```python
from build123d import *

# Parameters (mm, degrees)
SKETCH1_W            = 208
SKETCH1_H            = 128
SKETCH1_W_2          = 200
SKETCH1_H_2          = 120
SKETCH1_W_3          = 8
SKETCH1_H_3          = 8
BOSS_EXTRUDE1_DEPTH  = 16
SKETCH1_3_W          = 208
SKETCH1_3_H          = 128
SKETCH1_3_R          = 8.4
BOSS_EXTRUDE2_DEPTH  = 4
M4_CLEARANCE_HOLE1_D = 4.8
FILLET2_R            = 8
FILLET1_R            = 4
FILLET3_R            = 8
FILLET4_R            = 3
SKETCH8_R            = 4.25
CUT_EXTRUDE1_DEPTH   = 7


# Some blends are built 0.0001 mm under size
with BuildPart() as part:
    # Sketch1 → Boss-Extrude1 (new body)
    # profile 1 of 5: a face of its own
    with BuildSketch(Plane(origin=(0, 0, 0), x_dir=(1, 0, 0), z_dir=(0, 1, 0))):
        with Locations((100, 60)):
            Rectangle(SKETCH1_W, SKETCH1_H)
        with Locations((100, 60)):
            Rectangle(SKETCH1_W_2, SKETCH1_H_2, mode=Mode.SUBTRACT)
    # profile 2 of 5: a face of its own
    with BuildSketch(Plane(origin=(0, 0, 0), x_dir=(1, 0, 0), z_dir=(0, 1, 0))):
        with Locations((4, 4)):
            Rectangle(SKETCH1_W_3, SKETCH1_H_3)
    # profile 3 of 5: a face of its own
    with BuildSketch(Plane(origin=(0, 0, 0), x_dir=(1, 0, 0), z_dir=(0, 1, 0))):
        with Locations((196, 4)):
            Rectangle(SKETCH1_W_3, SKETCH1_H_3)
    # profile 4 of 5: a face of its own
    with BuildSketch(Plane(origin=(0, 0, 0), x_dir=(1, 0, 0), z_dir=(0, 1, 0))):
        with Locations((196, 116)):
            Rectangle(SKETCH1_W_3, SKETCH1_H_3)
    # profile 5 of 5: a face of its own
    with BuildSketch(Plane(origin=(0, 0, 0), x_dir=(1, 0, 0), z_dir=(0, 1, 0))):
        with Locations((4, 116)):
            Rectangle(SKETCH1_W_3, SKETCH1_H_3)
    extrude(amount=-BOSS_EXTRUDE1_DEPTH)

    # Sketch1<3> → Boss-Extrude2 (add)
    with BuildSketch(Plane(origin=(0, 0, 0), x_dir=(1, 0, 0), z_dir=(0, 1, 0))):
        with Locations((100, 60)):
            Rectangle(SKETCH1_3_W, SKETCH1_3_H)
        with Locations(Location((85, 90, 0), (0, 0, 270))):
            Circle(SKETCH1_3_R, mode=Mode.SUBTRACT)
        with Locations(Location((19.5, 100.5, 0), (0, 0, 270))):
            Circle(SKETCH1_3_R, mode=Mode.SUBTRACT)
        with Locations(Location((19.5, 19.5, 0), (0, 0, 270))):
            Circle(SKETCH1_3_R, mode=Mode.SUBTRACT)
        with Locations(Location((19.5, 46.5, 0), (0, 0, 270))):
            Circle(SKETCH1_3_R, mode=Mode.SUBTRACT)
        with Locations(Location((85, 30, 0), (0, 0, 270))):
            Circle(SKETCH1_3_R, mode=Mode.SUBTRACT)
        with Locations(Location((85, 60, 0), (0, 0, 270))):
            Circle(SKETCH1_3_R, mode=Mode.SUBTRACT)
        with Locations(Location((149, 19.5, 0), (0, 0, 270))):
            Circle(SKETCH1_3_R, mode=Mode.SUBTRACT)
        with Locations(Location((181, 19.5, 0), (0, 0, 270))):
            Circle(SKETCH1_3_R, mode=Mode.SUBTRACT)
        with BuildLine():
            ThreePointArc((163.25, 48.633932078), (153.5, 60), (163.25, 71.366067922))
            Line((163.25, 71.366067922), (163.25, 72.25))
            ThreePointArc((163.25, 72.25), (165, 74), (166.75, 72.25))
            Line((166.75, 72.25), (166.75, 71.366067922))
            ThreePointArc((166.75, 71.366067922), (176.5, 60), (166.75, 48.633932078))
            Line((166.75, 48.633932078), (166.75, 47.75))
            ThreePointArc((166.75, 47.75), (165, 46), (163.25, 47.75))
            Line((163.25, 47.75), (163.25, 48.633932078))
        make_face(mode=Mode.SUBTRACT)
        with Locations(Location((19.5, 73.5, 0), (0, 0, 270))):
            Circle(SKETCH1_3_R, mode=Mode.SUBTRACT)
    extrude(amount=BOSS_EXTRUDE2_DEPTH)

    # M4 Clearance Hole1 (through all)
    with Locations(Plane(origin=(0, 4, 0), x_dir=(1, 0, 0), z_dir=(0, 1, 0))):
        with Locations((3, 117), (197, 3), (3, 3), (197, 117)):
            Hole(M4_CLEARANCE_HOLE1_D / 2)

    # Fillet2
    fillet2_edges = [part.edges().sort_by_distance(p)[0] for p in [
        (204, -6, 4),
        (-4, -6, 4),
        (-4, -6, -124),
        (204, -6, -124),
    ]]
    fillet(fillet2_edges, radius=FILLET2_R)

    # Fillet1
    fillet1_edges = [part.edges().sort_by_distance(p)[0] for p in [
        (192, -8, 0),
        (192, -8, -8),
        (200, -8, -8),
        (8, -8, 0),
        (8, -8, -8),
        (0, -8, -8),
        (0, -8, -112),
        (8, -8, -120),
        (8, -8, -112),
        (192, -8, -120),
        (192, -8, -112),
        (200, -8, -112),
    ]]
    fillet(fillet1_edges, radius=FILLET1_R - 0.0001)  # a hair under: the kernel refuses the full size

    # Fillet3
    # the kernel refuses this fillet: 8 mm, written as the material it takes off along each edge
    with BuildSketch(Plane(origin=(-4, 4, -116), x_dir=(0, -1, 0), z_dir=(0, 0, 1)), Plane(origin=(204, 4, -4), x_dir=(0, -1, 0), z_dir=(0, 0, -1))) as fillet3_piece_1:
        with BuildLine():
            CenterArc((FILLET3_R, FILLET3_R), FILLET3_R, 180, 90)
            Line((0, FILLET3_R), (0, 0))
            Line((0, 0), (FILLET3_R, 0))
        make_face()
    extrude(amount=112, mode=Mode.SUBTRACT)
    with BuildSketch(Plane(origin=(196, 4, -124), x_dir=(0, -1, 0), z_dir=(-1, 0, 0)), Plane(origin=(4, 4, 4), x_dir=(0, -1, 0), z_dir=(1, 0, 0))) as fillet3_piece_2:
        with BuildLine():
            CenterArc((FILLET3_R, FILLET3_R), FILLET3_R, 180, 90)
            Line((0, FILLET3_R), (0, 0))
            Line((0, 0), (FILLET3_R, 0))
        make_face()
    extrude(amount=192, mode=Mode.SUBTRACT)
    with BuildSketch(Plane(origin=(4, 4, -4), x_dir=(0, 0, 1), z_dir=(1, 0, 0))) as fillet3_piece_3:
        with BuildLine():
            CenterArc((8 - FILLET3_R, FILLET3_R), FILLET3_R, 270, 90)
            Line((8 - FILLET3_R, 0), (8, 0))
            Line((8, 0), (8, FILLET3_R))
        make_face()
    revolve(axis=Axis((4, 4, -4), (0, -1, 0)), revolution_arc=90, mode=Mode.SUBTRACT)
    with BuildSketch(Plane(origin=(196, 4, -4), x_dir=(1, 0, 0), z_dir=(0, 0, -1))) as fillet3_piece_4:
        with BuildLine():
            CenterArc((8 - FILLET3_R, FILLET3_R), FILLET3_R, 270, 90)
            Line((8 - FILLET3_R, 0), (8, 0))
            Line((8, 0), (8, FILLET3_R))
        make_face()
    revolve(axis=Axis((196, 4, -4), (0, -1, 0)), revolution_arc=90, mode=Mode.SUBTRACT)
    with BuildSketch(Plane(origin=(196, 4, -116), x_dir=(1, 0, 0), z_dir=(0, 0, 1))) as fillet3_piece_5:
        with BuildLine():
            CenterArc((8 - FILLET3_R, -FILLET3_R), FILLET3_R, 0, 90)
            Line((8 - FILLET3_R, 0), (8, 0))
            Line((8, 0), (8, -FILLET3_R))
        make_face()
    revolve(axis=Axis((196, 4, -116), (0, 1, 0)), revolution_arc=90, mode=Mode.SUBTRACT)
    with BuildSketch(Plane(origin=(4, 4, -116), x_dir=(0, 0, -1), z_dir=(1, 0, 0))) as fillet3_piece_6:
        with BuildLine():
            CenterArc((8 - FILLET3_R, -FILLET3_R), FILLET3_R, 0, 90)
            Line((8 - FILLET3_R, 0), (8, 0))
            Line((8, 0), (8, -FILLET3_R))
        make_face()
    revolve(axis=Axis((4, 4, -116), (0, 1, 0)), revolution_arc=90, mode=Mode.SUBTRACT)

    # Fillet4
    fillet4_edges = [part.edges().sort_by_distance(p)[0] for p in [
        (200, 0, -60),
        (100, 0, 0),
        (0, 0, -60),
        (100, 0, -120),
        (198.828456414, 0, -110.828456414),
        (190.828456414, 0, -118.828456414),
        (9.171543586, 0, -118.828456414),
        (1.171543586, 0, -110.828456414),
        (1.171543586, 0, -9.171543586),
        (9.171543586, 0, -1.171543586),
        (198.828456414, 0, -9.171543586),
        (190.828456414, 0, -1.171543586),
        (193.171543586, 0, -6.828456414),
        (6.828456414, 0, -6.828456414),
        (6.828456414, 0, -113.171543586),
        (193.171543586, 0, -113.171543586),
    ]]
    fillet(fillet4_edges, radius=FILLET4_R)

    # Sketch8 → Cut-Extrude1 (cut)
    with BuildSketch(Plane(origin=(0, 4, 0), x_dir=(1, 0, 0), z_dir=(0, 1, 0))):
        with Locations(Location((3, 117, 0), (0, 0, 270))):
            Circle(SKETCH8_R)
        with Locations(Location((197, 117, 0), (0, 0, 270))):
            Circle(SKETCH8_R)
        with Locations(Location((197, 3, 0), (0, 0, 270))):
            Circle(SKETCH8_R)
        with Locations(Location((3, 3, 0), (0, 0, 270))):
            Circle(SKETCH8_R)
    extrude(amount=-CUT_EXTRUDE1_DEPTH, mode=Mode.SUBTRACT)


solid = part.part
```
Geometry check sheet. Reference: the model listing, model coordinates, mm. A direction names the side the tool comes from. Coordinates: 2 decimals unless noted, no trailing zeros. Order: outer loops, then holes, each group sorted by start corner. A loop starts at its lowest first (then second) coordinate and runs counter-clockwise, first axis right, second up. Notation, with made-up numbers: M 18,57.25 L 25,57.25 A25 ccw 25,71.25 Z; hole C 77,51.25 d9. An arc over 180 degrees is marked long. One line per question, with ' | ' between items. Start each with the question number.
Item 1: Cross-section at C-C on x = 85. Enter the section's corners in (y, z).
Item 2: Set-up check for faces 1 (the cylindrical face through (153.5, 2, -59.8)), 2 (the cylindrical face through (-1.594, 1.719, -60.784)), 3 (the cylindrical face through (1.141, -9.591, -9.203)): record each of +Z, -Z, +X, -X, +Y, -Y from which the full face is reachable in a straight line by a thin tool's end or side.
Item 3: Cross-section at B-B on z = -90. Enter the section's corners in (x, y), then the cut area to 3 significant figures.
Item 4: Material ranges on L1, parallel to X at y = -9.5, z = -88.5; L2, parallel to Z at x = 158, y = -13.75; L3, parallel to Z at x = 3, y = 1, recorded low to high. Write a range as [from, to].
Item 5: Cross-section at A-A on x = 149. Enter the section's corners in (y, z), then the cut area to 3 significant figures.
Item 6: Cross-section at D-D on z = -60. Enter the section's corners in (x, y), then the cut area to 3 significant figures.
Item 7: Gauge pin test, flat ends, axial feed: pin 1 (8 mm diameter, centred on x = 126.5, z = -35, fed in from -Y); pin 2 (15 mm diameter, centred on x = 85, z = -90, fed in from -Y); pin 3 (10 mm diameter, centred on x = 176, y = 2, fed in from +Z); pin 4 (0.7 mm diameter, centred on y = 2.5, z = -48.5, fed in from -X). Record the tip position at first contact, or that the pin passes through.
Item 8: Draft check along X on faces 4 (the flat face through (99, -10, 4)), 5 (the cylindrical face through (-1.719, -9.916, 1.594)), 6 (the cylindrical face through (19.87, 1.97, -54.89)), 7 (the cylindrical face through (140.8, 1.97, -21.32)). Enter one of: pulls with the +X half, pulls with the -X half, needs draft (parallel to the pull), parting line crosses it, or undercut.
Findings:
1) outline: M -16,-124 L -4,-124 A8 ccw 4,-116 L 4,-98.4 L 0,-98.4 L 0,-117 A3 cw -3,-120 L -16,-120 Z; M -16,0 L -3,0 A3 cw 0,-3 L 0,-21.6 L 4,-21.6 L 4,-4 A8 ccw -4,4 L -16,4 Z; M 0,-81.6 L 4,-81.6 L 4,-68.4 L 0,-68.4 Z; M 0,-51.6 L 4,-51.6 L 4,-38.4 L 0,-38.4 Z
2) face 1: +Y, -Y | face 2: +Z, -Z, -X, +Y | face 3: -Y
3) outline: M -4,-16 L 0,-16 L 0,-3 A3 cw 3,0 L 76.6,0 L 76.6,4 L 4,4 A8 ccw -4,-4 Z; M 93.4,0 L 197,0 A3 cw 200,-3 L 200,-16 L 204,-16 L 204,-4 A8 ccw 196,4 L 93.4,4 Z | area: 869 mm²
4) L1: x = [-4, 0], [200, 204] | L2: z = [-124, -120], [0, 4] | L3: z = [-122.16, -121.25], [-112.75, -7.25], [1.25, 2.16]
5) outline: M -16,-124 L -4,-124 A8 ccw 4,-116 L 4,-27.9 L 0,-27.9 L 0,-117 A3 cw -3,-120 L -16,-120 Z; M -16,0 L -3,0 A3 cw 0,-3 L 0,-11.1 L 4,-11.1 L 4,-4 A8 ccw -4,4 L -16,4 Z | area: 549 mm²
6) outline: M -4,-16 L 0,-16 L 0,-3 A3 cw 3,0 L 76.6,0 L 76.6,4 L 4,4 A8 ccw -4,-4 Z; M 93.4,0 L 153.5,0 L 153.5,4 L 93.4,4 Z; M 176.5,0 L 197,0 A3 cw 200,-3 L 200,-16 L 204,-16 L 204,-4 A8 ccw 196,4 L 176.5,4 Z | area: 777 mm²
7) pin 1: stops at y = 0 | pin 2: passes through | pin 3: stops at z = 3.94 | pin 4: stops at x = -1.12
8) face 4: needs draft | face 5: pulls with the -X half | face 6: undercut | face 7: undercut
